The listing builds one solid part. Answer for the finished solid, in the listing's coordinates (mm). A direction names the side the tool comes from. Coordinates: 2 decimals unless noted, no trailing zeros. Write each loop counter-clockwise with the first axis right and the second up, starting at its lowest first coordinate (ties: lowest second). Pieces come first, ordered by that corner, then holes.
(1) The part is cut by section D-D on z = 1.75. Give the number of separate pieces and of enclosed holes in the cut face, plus the area to 3 significant figures.
(2) Given P1, Ø2, axis at x = 11.5, z = -1.5, coming from the +Y side; P2, Ø0.9, axis at y = 1.5, z = -1.5, coming from the -X side; P3, Ø5, axis at x = 9.5, y = 1.5, coming from the -Z side, each flat-ended and moving along its own axis, determine where each tip first touches the part or whether it passes through.
(3) The part is cut by section B-B on x = 21.5. Determine the outline of the cut face in (y, z).
(4) For a pull along Y with two mould halves and no side action, classify faces 4 (the flat face through (14, 5, 2)), 5 (the flat face through (23, 3.25, 0)), 6 (the flat face through (9, 0, 0)) as +Y half, -Y half, draft (parallel to the pull), parting line (faces both ways), or undercut.
(5) Which of the six approach directions +Z, -Z, +X, -X, +Y, -Y give full straight-line access (tool end or side, diameter ignored) to faces 1 (the flat face through (18, 0, -1)), 2 (the flat face through (19.597, -0.07, -3)), 3 (the flat face through (26.25, 0, 0))?
(6) Straight lines are drawn through the part: line 1 (X direction, y = -1.25, z = -1.75); line 2 (Y direction, x = 5.75, z = 3.75); line 3 (X direction, y = 0.75, z = 0.5). For each, find the intervals that lie inside material, in ascending order.
(7) The part is cut by section C-C on y = 3.75. Determine the outline of the cut face in (x, z).
(8) The part is cut by section A-A on z = -1.5. Determine the outline of the cut face in (x, y).
from build123d import *

# Parameters (mm, degrees)
F0_W     = 28
F0_H     = 10
F1_DEPTH = 5
F3_DEPTH = 6
F4_W     = 10
F4_H     = 10
F5_DEPTH = 3
F6_W     = 6.5
F6_H     = 6.5
F7_DEPTH = 6


with BuildPart() as f1:
    # F0 (on Top) → F1 (new body)
    with BuildSketch(Plane.XY):
        with Locations((14, 0)):
            Rectangle(F0_W, F0_H)
    extrude(amount=F1_DEPTH)

    # F2 (on face) → F3 (cut)
    with BuildSketch(Plane.XY.offset(5)):
        with BuildLine():
            Line((7.9837568295, 0.2543793255), (8.7316052217, 0.3175419863))
            ThreePointArc((8.7316052217, 0.3175419863), (8.5841547072, 0.9405553941), (8.2966430552, 1.512590717))
            Line((8.2966430552, 1.512590717), (7.6831577744, 1.0802684419))
            ThreePointArc((7.6831577744, 1.0802684419), (7.8793852416, 0.6840402867), (7.9837568295, 0.2543793255))
        make_face()
        with BuildLine():
            Line((7.9837568295, -0.2543793255), (7.9837568295, 0.2543793255))
            ThreePointArc((7.9837568295, 0.2543793255), (7.8793852416, 0.6840402867), (7.6831577744, 1.0802684419))
            Line((7.6831577744, 1.0802684419), (7.3561340172, 1.4700001794))
            ThreePointArc((7.3561340172, 1.4700001794), (7, 1.7320508076), (6.5949904904, 1.9094465995))
            Line((6.5949904904, 1.9094465995), (6.0939610264, 1.9977916121))
            ThreePointArc((6.0939610264, 1.9977916121), (5.6527036447, 1.969615506), (5.2284205433, 1.8451734721))
            Line((5.2284205433, 1.8451734721), (4.7878226271, 1.5907941466))
            ThreePointArc((4.7878226271, 1.5907941466), (4.4679111138, 1.2855752194), (4.2228811992, 0.9175231702))
            Line((4.2228811992, 0.9175231702), (4.0488754925, 0.4394464201))
            ThreePointArc((4.0488754925, 0.4394464201), (4, 0), (4.0488754925, -0.4394464201))
            Line((4.0488754925, -0.4394464201), (4.2228811992, -0.9175231702))
            ThreePointArc((4.2228811992, -0.9175231702), (4.4679111138, -1.2855752194), (4.7878226271, -1.5907941466))
            Line((4.7878226271, -1.5907941466), (5.2284205433, -1.8451734721))
            ThreePointArc((5.2284205433, -1.8451734721), (5.6527036447, -1.969615506), (6.0939610264, -1.9977916121))
            Line((6.0939610264, -1.9977916121), (6.5949904904, -1.9094465995))
            ThreePointArc((6.5949904904, -1.9094465995), (7, -1.7320508076), (7.3561340172, -1.4700001794))
            Line((7.3561340172, -1.4700001794), (7.6831577744, -1.0802684419))
            ThreePointArc((7.6831577744, -1.0802684419), (7.8793852416, -0.6840402867), (7.9837568295, -0.2543793255))
        make_face()
        with BuildLine():
            ThreePointArc((8, 0), (7.9959350765, 0.1274486974), (7.9837568295, 0.2543793255))
            Line((7.9837568295, 0.2543793255), (7.9837568295, -0.2543793255))
            ThreePointArc((7.9837568295, -0.2543793255), (7.9959350765, -0.1274486974), (8, 0))
        make_face()
        with BuildLine():
            Line((7.3561340172, 1.4700001794), (7.6831577744, 1.0802684419))
            ThreePointArc((7.6831577744, 1.0802684419), (7.5320888862, 1.2855752194), (7.3561340172, 1.4700001794))
        make_face()
        with BuildLine():
            Line((8.7316052217, -0.3175419863), (7.9837568295, -0.2543793255))
            ThreePointArc((7.9837568295, -0.2543793255), (7.8793852416, -0.6840402867), (7.6831577744, -1.0802684419))
            Line((7.6831577744, -1.0802684419), (8.2966430552, -1.512590717))
            ThreePointArc((8.2966430552, -1.512590717), (8.5841547072, -0.9405553941), (8.7316052217, -0.3175419863))
        make_face()
        with BuildLine():
            ThreePointArc((6.5949904904, 1.9094465995), (7, 1.7320508076), (7.3561340172, 1.4700001794))
            Line((7.3561340172, 1.4700001794), (7.8884189465, 1.9990932651))
            ThreePointArc((7.8884189465, 1.9990932651), (7.375, 2.3815698604), (6.7870560788, 2.6349654132))
            Line((6.7870560788, 2.6349654132), (6.5949904904, 1.9094465995))
        make_face()
        with BuildLine():
            ThreePointArc((7.3561340172, -1.4700001794), (7.5320888862, -1.2855752194), (7.6831577744, -1.0802684419))
            Line((7.6831577744, -1.0802684419), (7.3561340172, -1.4700001794))
        make_face()
        with BuildLine():
            Line((6.0939610264, 1.9977916121), (6.5949904904, 1.9094465995))
            ThreePointArc((6.5949904904, 1.9094465995), (6.3472963553, 1.969615506), (6.0939610264, 1.9977916121))
        make_face()
        with BuildLine():
            Line((7.8884189465, -1.9990932651), (7.3561340172, -1.4700001794))
            ThreePointArc((7.3561340172, -1.4700001794), (7, -1.7320508076), (6.5949904904, -1.9094465995))
            Line((6.5949904904, -1.9094465995), (6.7870560788, -2.6349654132))
            ThreePointArc((6.7870560788, -2.6349654132), (7.375, -2.3815698604), (7.8884189465, -1.9990932651))
        make_face()
        with BuildLine():
            ThreePointArc((5.2284205433, 1.8451734721), (5.6527036447, 1.969615506), (6.0939610264, 1.9977916121))
            Line((6.0939610264, 1.9977916121), (6.1616204589, 2.7452465877))
            ThreePointArc((6.1616204589, 2.7452465877), (5.5224675114, 2.7082213208), (4.9091968161, 2.5244105082))
            Line((4.9091968161, 2.5244105082), (5.2284205433, 1.8451734721))
        make_face()
        with BuildLine():
            ThreePointArc((6.0939610264, -1.9977916121), (6.3472963553, -1.969615506), (6.5949904904, -1.9094465995))
            Line((6.5949904904, -1.9094465995), (6.0939610264, -1.9977916121))
        make_face()
        with BuildLine():
            Line((4.7878226271, 1.5907941466), (5.2284205433, 1.8451734721))
            ThreePointArc((5.2284205433, 1.8451734721), (5, 1.7320508076), (4.7878226271, 1.5907941466))
        make_face()
        with BuildLine():
            Line((6.1616204589, -2.7452465877), (6.0939610264, -1.9977916121))
            ThreePointArc((6.0939610264, -1.9977916121), (5.6527036447, -1.969615506), (5.2284205433, -1.8451734721))
            Line((5.2284205433, -1.8451734721), (4.9091968161, -2.5244105082))
            ThreePointArc((4.9091968161, -2.5244105082), (5.5224675114, -2.7082213208), (6.1616204589, -2.7452465877))
        make_face()
        with BuildLine():
            ThreePointArc((4.2228811992, 0.9175231702), (4.4679111138, 1.2855752194), (4.7878226271, 1.5907941466))
            Line((4.7878226271, 1.5907941466), (4.3591979623, 2.2068685219))
            ThreePointArc((4.3591979623, 2.2068685219), (3.8933777814, 1.7676659266), (3.541736486, 1.2326558707))
            Line((3.541736486, 1.2326558707), (4.2228811992, 0.9175231702))
        make_face()
        with BuildLine():
            ThreePointArc((4.7878226271, -1.5907941466), (5, -1.7320508076), (5.2284205433, -1.8451734721))
            Line((5.2284205433, -1.8451734721), (4.7878226271, -1.5907941466))
        make_face()
        with BuildLine():
            Line((4.0488754925, 0.4394464201), (4.2228811992, 0.9175231702))
            ThreePointArc((4.2228811992, 0.9175231702), (4.1206147584, 0.6840402867), (4.0488754925, 0.4394464201))
        make_face()
        with BuildLine():
            Line((4.3591979623, -2.2068685219), (4.7878226271, -1.5907941466))
            ThreePointArc((4.7878226271, -1.5907941466), (4.4679111138, -1.2855752194), (4.2228811992, -0.9175231702))
            Line((4.2228811992, -0.9175231702), (3.541736486, -1.2326558707))
            ThreePointArc((3.541736486, -1.2326558707), (3.8933777814, -1.7676659266), (4.3591979623, -2.2068685219))
        make_face()
        with BuildLine():
            ThreePointArc((4.0488754925, -0.4394464201), (4, 0), (4.0488754925, 0.4394464201))
            Line((4.0488754925, 0.4394464201), (3.3245249747, 0.6358721481))
            ThreePointArc((3.3245249747, 0.6358721481), (3.25, 0), (3.3245249747, -0.6358721481))
            Line((3.3245249747, -0.6358721481), (4.0488754925, -0.4394464201))
        make_face()
        with BuildLine():
            ThreePointArc((4.0488754925, -0.4394464201), (4.1206147584, -0.6840402867), (4.2228811992, -0.9175231702))
            Line((4.2228811992, -0.9175231702), (4.0488754925, -0.4394464201))
        make_face()
    extrude(amount=-F3_DEPTH, mode=Mode.SUBTRACT)

    # F4 (on face) → F5 (join)
    with BuildSketch(Plane(origin=(0, 0, 0), x_dir=(1, 0, 0), z_dir=(0, 0, -1))):
        with Locations((23, 0)):
            Rectangle(F4_W, F4_H)
    extrude(amount=F5_DEPTH)

    # F6 (on face) → F7 (cut)
    with BuildSketch(Plane(origin=(0, 0, -3), x_dir=(1, 0, 0), z_dir=(0, 0, -1))):
        with Locations((23, 0)):
            Rectangle(F6_W, F6_H)
    extrude(amount=-F7_DEPTH, mode=Mode.SUBTRACT)


solid = f1.part
Model answer:
1. separate pieces: 1
1. enclosed holes: 2
1. area: 218 mm2
2. P1: passes through
2. P2: stops at x = 18
2. P3: stops at z = 0
3. outline: (-5, -3) - (-3.25, -3) - (-3.25, 3) - (3.25, 3) - (3.25, -3) - (5, -3) - (5, 5) - (-5, 5) - close
4. face 4: +Y half
4. face 5: undercut
4. face 6: draft
5. face 1: -Z, -X, +Y, -Y
5. face 2: -Z, +X, -X, +Y, -Y
5. face 3: -Z
6. line 1: x = 18 to 19.75, 26.25 to 28
6. line 2: y = -5 to -2.74, 2.74 to 5
6. line 3: x = 0 to 4.15, 8.65 to 19.75, 26.25 to 28
7. outline: (0, 0) - (18, 0) - (18, -3) - (28, -3) - (28, 5) - (0, 5) - close
8. outline: (18, -5) - (28, -5) - (28, 5) - (18, 5) - close; hole (19.75, -3.25) - (26.25, -3.25) - (26.25, 3.25) - (19.75, 3.25) - close
